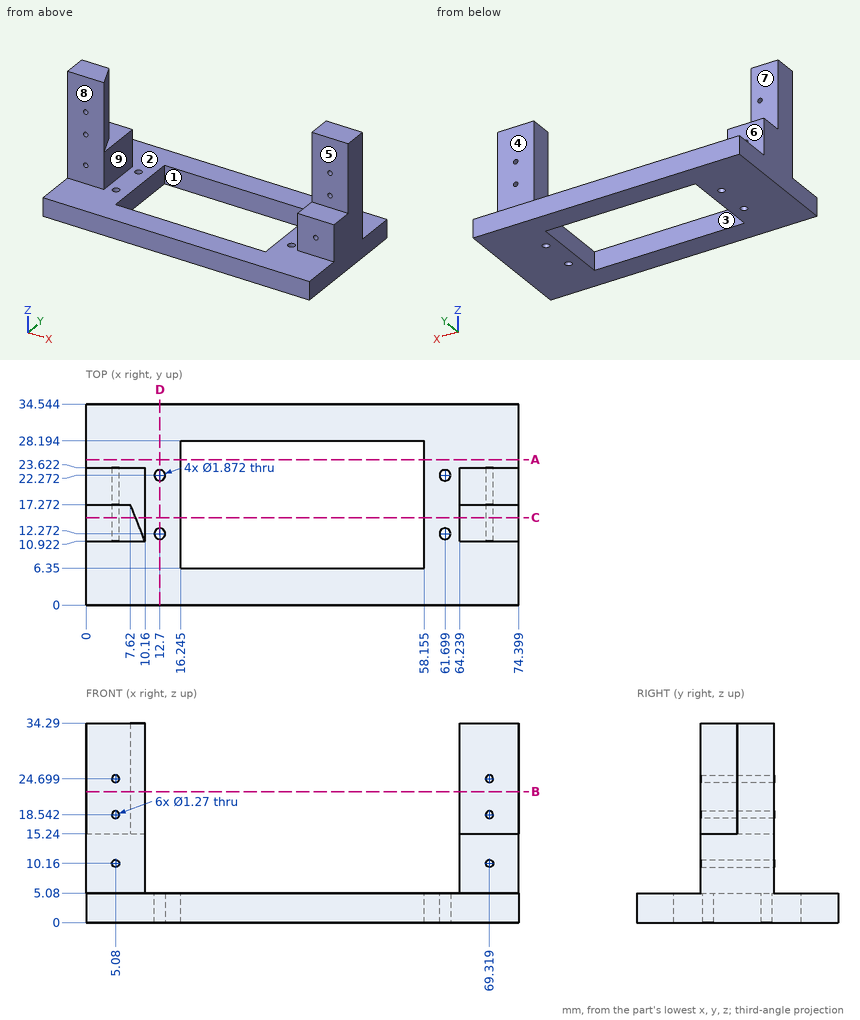
Source: three-view drawing plus pictorial views. Frame: mm from the lowest corner of the part. A direction names the side the tool comes from. Round coordinates to 2 decimals unless told otherwise and drop trailing zeros. Write each loop counter-clockwise with the first axis right and the second up, starting at its lowest first coordinate (ties: lowest second). Pieces come first, ordered by that corner, then holes. Notation, with made-up numbers: (15.25, 36) -> (23.25, 36) arc R15 ccw to (23.25, 43) -> close; hole circle Ø10 at (-7.75, -19). An arc over 180 degrees is marked (long way). Return JSON: item names as keys, results as strings.
Q1. Section C-C on y = 15. Return the cut outline in (x, z) (1 decimal), and give its area (3 significant figures).
From the geometry:
{"outline": "(0, 0) -> (16.2, 0) -> (16.2, 5.1) -> (10.2, 5.1) -> (10.2, 15.2) -> (8.5, 15.2) -> (8.5, 34.3) -> (0, 34.3) -> close; (58.2, 0) -> (74.4, 0) -> (74.4, 15.2) -> (64.2, 15.2) -> (64.2, 5.1) -> (58.2, 5.1) -> close; hole circle Ø1.3 at (5.1, 10.2); hole circle Ø1.3 at (5.1, 18.5); hole circle Ø1.3 at (5.1, 24.7); hole circle Ø1.3 at (69.3, 10.2)", "area": "529 mm2"}
Q2. Ray query, line 1 (Y direction, x = 12.7, z = 2.7); line 2 (Y direction, x = 45, z = 2.5); line 3 (Z direction, x = 5.08, y = 19.5) (1 decimal). Return the intervals inside material, ascending.
From the geometry:
{"line 1": "0 to 11.34, 13.21 to 21.34, 23.21 to 34.54", "line 2": "0 to 6.35, 28.19 to 34.54", "line 3": "0 to 9.5, 10.8 to 15.2"}
Q3. First-contact query: pin 1 Ø5 at (x, y) = (67.5, 15.5) entering from +Z; pin 2 Ø8 at (x, y) = (10.5, 27.5) entering from +Z; pin 3 Ø8 at (x, z) = (4, 25) entering from -Y; pin 4 Ø2 at (x, z) = (5.08, 18.542) entering from +Y. Flat tips, straight axial feed; report the tip coordinate or a pass-through.
From the geometry:
{"pin 1": "z = 34.29", "pin 2": "z = 15.24", "pin 3": "y = 10.92", "pin 4": "y = 17.27"}
Q4. Mould query, pull axis Y, two halves, no side actions, for the marked faces 1, 2, 3 and 4. Classes: +Y half, -Y half, draft (parallel to the pull), parting line (faces both ways), or undercut.
From the geometry:
{"face 1": "undercut", "face 2": "draft", "face 3": "undercut", "face 4": "+Y half"}
Q5. Set-up query: the marked faces 5, 6, 7, 8 and 9. Return all of +Z, -Z, +X, -X, +Y, -Y with unobstructed straight access to the full face (end or side cutting, diameter ignored); none if empty.
From the geometry:
{"face 5": "+Z, +X, -Y", "face 6": "+Z, +X, -X, +Y", "face 7": "+Z, -X, +Y", "face 8": "+Z, +X, -X, -Y", "face 9": "+Z, +Y, -Y"}
Q6. Section A-A on y = 25. Return the cut outline in (x, z) (1 decimal).
From the geometry:
{"outline": "(0, 0) -> (16.2, 0) -> (16.2, 5.1) -> (0, 5.1) -> close; (58.2, 0) -> (74.4, 0) -> (74.4, 5.1) -> (58.2, 5.1) -> close"}
Q7. Section D-D on x = 12.7. Return the cut outline in (y, z).
From the geometry:
{"outline": "(0, 0) -> (11.34, 0) -> (11.34, 5.08) -> (0, 5.08) -> close; (13.21, 0) -> (21.34, 0) -> (21.34, 5.08) -> (13.21, 5.08) -> close; (23.21, 0) -> (34.54, 0) -> (34.54, 5.08) -> (23.21, 5.08) -> close"}
Q8. Section B-B on z = 22.5. Return the cut outline in (x, y).
From the geometry:
{"outline": "(0, 10.92) -> (10.16, 10.92) -> (7.62, 17.27) -> (0, 17.27) -> close; (64.24, 17.27) -> (74.4, 17.27) -> (74.4, 23.62) -> (64.24, 23.62) -> close"}
